Read the model definition and answer for the solid it produces. Units are mm, in the model's axes. Face numbers are marked on the shaded views. A direction names the side the tool comes from. Round coordinates to 2 decimals unless told otherwise and drop trailing zeros. Order: outer loops, then holes, each group sorted by start corner. A loop starts at its lowest first (then second) coordinate and runs counter-clockwise, first axis right, second up. Notation, with made-up numbers: (-40, 29.25) - (-12, 29.25) arc R11 cw to (-12, 44.25) - close; hole circle Ø1 at (41, 62). An arc over 180 degrees is marked (long way). Answer as a JSON object with one key per item and string values. Group by question number.
Q1. Given pin 1 Ø6 at (x, z) = (-6, 18.5) entering from +Y; pin 2 Ø3 at (y, z) = (-2.5, 51) entering from -X; pin 3 Ø4 at (x, z) = (-1, 39) entering from -Y; pin 4 Ø10 at (x, y) = (-10, 4) entering from +Z, each flat-ended and moving along its own axis, determine where each tip first touches the part or whether it passes through.
Q2. Consider line 1 (Y direction, x = 3.5, z = 55); line 2 (Y direction, x = -1.5, z = 49.5); line 3 (X direction, y = -0.25, z = 19.5). Determine where each line is inside the solid, lowest interval first.
Q3. A cutting plane is placed at C-C on z = 25. Determine the outline of the cut face in (x, y).
Q4. A tool of negligible diameter and unlimited length cuts with its end or side. For the marked faces 5, 6, 7 and 8, from which of +Z, -Z, +X, -X, +Y, -Y can it reach the whole face along a straight path? Write none if from no direction.
Q5. A cutting plane is placed at D-D on z = 70. Determine the outline of the cut face in (x, y), and give its area (3 significant figures).
Q6. A cutting plane is placed at B-B on y = -7.75. Determine the outline of the cut face in (x, z).
Q7. The mould has two halves that part along X. Classify the marked faces 1, 2, 3 and 4: pulls with the +X half, pulls with the -X half, needs draft (parallel to the pull), parting line crosses it, or undercut.
Q8. A cutting plane is placed at A-A on x = 2.5. Determine the outline of the cut face in (y, z), and give its area (3 significant figures).
```python
from build123d import *

# Parameters (mm, degrees)
F0_R      = 11.5
F0_R_2    = 6.5
F1_DEPTH  = 75
F2_W      = 40
F2_H      = 22.7775762856
F3_DEPTH  = 75
F5_DEPTH  = 75
F7_DEPTH  = 75
F10_DEPTH = 15
F12_DEPTH = 10


# Not quite as in the source:
# - after a boolean that leaves OpenCascade's solid faulty, fix() repairs it


with BuildPart() as f1:
    # F0 (on Top) → F1 (new body)
    with BuildSketch(Plane.XY):
        Circle(F0_R)
        Circle(F0_R_2, mode=Mode.SUBTRACT)
    extrude(amount=F1_DEPTH)

    # F2 (on face) → F3 (cut, through all)
    with BuildSketch(Plane.XY.offset(75)):
        with Locations((0, -21.0887881428)):
            Rectangle(F2_W, F2_H)
        Polygon((-20, 9.7), (20, 9.7), (20, 33.5304923356), (-20, 28.7892241031), align=None)
    extrude(amount=-F3_DEPTH, mode=Mode.SUBTRACT)

    # F4 (on face) → F5 (join)
    with BuildSketch(Plane.XY.offset(75)):
        with BuildLine():
            Line((6.4621977686, 10.7), (-6.4621977686, 10.7))
            ThreePointArc((-6.4621977686, 10.7), (-12.5, 0), (-6.4621977686, -10.7))
            Line((-6.4621977686, -10.7), (6.4621977686, -10.7))
            ThreePointArc((6.4621977686, -10.7), (12.5, 0), (6.4621977686, 10.7))
        make_face()
        with BuildLine():
            ThreePointArc((-6.1773780846, -9.7), (-11.5, 0), (-6.1773780846, 9.7))
            Line((-6.1773780846, 9.7), (6.1773780846, 9.7))
            ThreePointArc((6.1773780846, 9.7), (11.5, 0), (6.1773780846, -9.7))
            Line((6.1773780846, -9.7), (-6.1773780846, -9.7))
        make_face(mode=Mode.SUBTRACT)
    extrude(amount=-F5_DEPTH)

    # F6 (on face) → F7 (cut)
    with BuildSketch(Plane.XY.offset(75)):
        with BuildLine():
            Line((-6.1773780846, -9.7), (6.1773780846, -9.7))
            ThreePointArc((6.1773780846, -9.7), (11.5, 0), (6.1773780846, 9.7))
            Line((6.1773780846, 9.7), (-6.1773780846, 9.7))
            ThreePointArc((-6.1773780846, 9.7), (-11.5, 0), (-6.1773780846, -9.7))
        make_face()
    extrude(amount=-F7_DEPTH, mode=Mode.SUBTRACT)

    # F9 (on mid) → F10 (join, symmetric)
    with BuildSketch(Plane.XY.offset(37.5)):
        with BuildLine():
            Line((5.6665686266, 11.7), (-5.6665686266, 11.7))
            ThreePointArc((-5.6665686266, 11.7), (-13, 0), (-5.6665686266, -11.7))
            Line((-5.6665686266, -11.7), (5.6665686266, -11.7))
            ThreePointArc((5.6665686266, -11.7), (13, 0), (5.6665686266, 11.7))
        make_face()
        with BuildLine():
            ThreePointArc((-6.1773780846, -9.7), (-11.5, 0), (-6.1773780846, 9.7))
            Line((-6.1773780846, 9.7), (6.1773780846, 9.7))
            ThreePointArc((6.1773780846, 9.7), (11.5, 0), (6.1773780846, -9.7))
            Line((6.1773780846, -9.7), (-6.1773780846, -9.7))
        make_face(mode=Mode.SUBTRACT)
    extrude(amount=F10_DEPTH, both=True)

    add(f1.part.fix(), mode=Mode.REPLACE)

    # F11 (on mid) → F12 (cut, symmetric)
    with BuildSketch(Plane.XY.offset(37.5)):
        with BuildLine():
            Line((-5.6665686266, -11.7), (5.6665686266, -11.7))
            ThreePointArc((5.6665686266, -11.7), (13, 0), (5.6665686266, 11.7))
            Line((5.6665686266, 11.7), (-5.6665686266, 11.7))
            ThreePointArc((-5.6665686266, 11.7), (-13, 0), (-5.6665686266, -11.7))
        make_face()
        with BuildLine():
            ThreePointArc((6.4621977686, 10.7), (12.5, 0), (6.4621977686, -10.7))
            Line((6.4621977686, -10.7), (-6.4621977686, -10.7))
            ThreePointArc((-6.4621977686, -10.7), (-12.5, 0), (-6.4621977686, 10.7))
            Line((-6.4621977686, 10.7), (6.4621977686, 10.7))
        make_face(mode=Mode.SUBTRACT)
    extrude(amount=F12_DEPTH, both=True, mode=Mode.SUBTRACT)

    add(f1.part.fix(), mode=Mode.REPLACE)


solid = f1.part
```
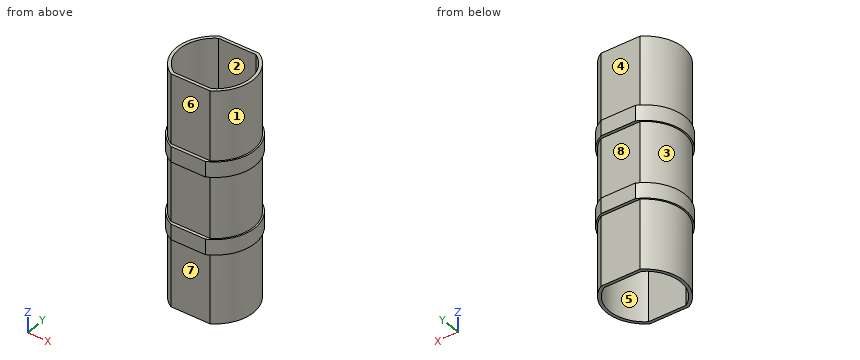
Result set:
{
 "1": {"pin 1": "stops at y = 10.7", "pin 2": "stops at x = -12.96", "pin 3": "stops at y = -10.7", "pin 4": "stops at z = 75"},
 "2": {"line 1": "y = -10.7 to -9.7, 9.7 to 10.7", "line 2": "y = -11.7 to -9.7, 9.7 to 11.7", "line 3": "x = -12.5 to -11.5, 11.5 to 12.5"},
 "3": {"outline": "(-5.67, -11.7) - (5.67, -11.7) arc R13 ccw to (5.67, 11.7) - (-5.67, 11.7) arc R13 ccw to start; hole (-6.18, -9.7) - (6.18, -9.7) arc R11.5 ccw to (6.18, 9.7) - (-6.18, 9.7) arc R11.5 ccw to start"},
 "4": {"face 5": "+Z, -Z", "face 6": "+Z, +X, -X, -Y", "face 7": "-Z, +X, -X, -Y", "face 8": "+X, -X, +Y"},
 "5": {"outline": "(-6.46, -10.7) - (6.46, -10.7) arc R12.5 ccw to (6.46, 10.7) - (-6.46, 10.7) arc R12.5 ccw to start; hole (-6.18, -9.7) - (6.18, -9.7) arc R11.5 ccw to (6.18, 9.7) - (-6.18, 9.7) arc R11.5 ccw to start", "area": "74.1 mm²"},
 "6": {"outline": "(-10.44, 22.5) - (-9.81, 22.5) - (-9.81, 0) - (-8.5, 0) - (-8.5, 75) - (-9.81, 75) - (-9.81, 52.5) - (-10.44, 52.5) - (-10.44, 47.5) - (-9.81, 47.5) - (-9.81, 27.5) - (-10.44, 27.5) - close; (8.5, 0) - (9.81, 0) - (9.81, 22.5) - (10.44, 22.5) - (10.44, 27.5) - (9.81, 27.5) - (9.81, 47.5) - (10.44, 47.5) - (10.44, 52.5) - (9.81, 52.5) - (9.81, 75) - (8.5, 75) - close"},
 "7": {"face 1": "pulls with the +X half", "face 2": "undercut", "face 3": "pulls with the -X half", "face 4": "needs draft"},
 "8": {"outline": "(-11.7, 22.5) - (-10.7, 22.5) - (-10.7, 0) - (-9.7, 0) - (-9.7, 75) - (-10.7, 75) - (-10.7, 52.5) - (-11.7, 52.5) - (-11.7, 47.5) - (-10.7, 47.5) - (-10.7, 27.5) - (-11.7, 27.5) - close; (9.7, 0) - (10.7, 0) - (10.7, 22.5) - (11.7, 22.5) - (11.7, 27.5) - (10.7, 27.5) - (10.7, 47.5) - (11.7, 47.5) - (11.7, 52.5) - (10.7, 52.5) - (10.7, 75) - (9.7, 75) - close", "area": "170 mm²"}
}
